```python
from build123d import *

# Parameters (mm, degrees)
SKETCH_1_W               = 764
SKETCH_1_H               = 1500
SKETCH_1_W_2             = 584
SKETCH_1_H_2             = 1320
EXTRUDE_1_DEPTH          = 18
SKETCH_1_3_W             = 28
SKETCH_1_3_H             = 60
EXTRUDE_2_DEPTH          = 18
PATTERN_LINEAR_1_COUNT   = 5
PATTERN_LINEAR_1_PITCH   = 250
MIRROR_1_COPY_1_SKETCH_W = 28
MIRROR_1_COPY_1_SKETCH_H = 60
MIRROR_1_COPY_1_DEPTH    = 18
MIRROR_1_COPY_2_SKETCH_W = 28
MIRROR_1_COPY_2_SKETCH_H = 60
MIRROR_1_COPY_2_DEPTH    = 18
MIRROR_1_COPY_3_SKETCH_W = 28
MIRROR_1_COPY_3_SKETCH_H = 60
MIRROR_1_COPY_3_DEPTH    = 18
MIRROR_1_COPY_4_SKETCH_W = 28
MIRROR_1_COPY_4_SKETCH_H = 60
MIRROR_1_COPY_4_DEPTH    = 18
SKETCH_1_4_W             = 62
SKETCH_1_4_H             = 20
CUT_EXTRUDE_1_DEPTH      = 855.940933632
PATTERN_LINEAR_2_COUNT   = 3
PATTERN_LINEAR_2_PITCH   = 250
MIRROR_2_COPY_1_SKETCH_W = 62
MIRROR_2_COPY_1_SKETCH_H = 20
MIRROR_2_COPY_1_DEPTH    = 855.940933632
MIRROR_2_COPY_2_SKETCH_W = 62
MIRROR_2_COPY_2_SKETCH_H = 20
MIRROR_2_COPY_2_DEPTH    = 855.940933632
FILLET_1_R               = 25
FILLET_2_R               = 25


with BuildPart() as part:
    # 草图1 → 凸台-拉伸1 (new body)
    with BuildSketch(Plane(origin=(0, 0, 0), x_dir=(1, 0, 0), z_dir=(0, 1, 0))):
        Rectangle(SKETCH_1_W, SKETCH_1_H)
        Rectangle(SKETCH_1_W_2, SKETCH_1_H_2, mode=Mode.SUBTRACT)
    extrude(amount=EXTRUDE_1_DEPTH)

    # 草图1<3> → 凸台-拉伸2 (add)
    with BuildSketch(Plane(origin=(0, 0, 0), x_dir=(1, 0, 0), z_dir=(0, 1, 0))):
        with Locations((-396, -500)):
            Rectangle(SKETCH_1_3_W, SKETCH_1_3_H)
    extrude_2 = extrude(amount=EXTRUDE_2_DEPTH)

    # 阵列(线性)1: 凸台-拉伸2 ×5
    with Locations(*[(0, 0, -i * PATTERN_LINEAR_1_PITCH) for i in range(1, PATTERN_LINEAR_1_COUNT)]):
        add(extrude_2)

    # 镜向1: 凸台-拉伸2 across plane
    add(extrude_2.mirror(Plane(origin=(0, 0, 0), x_dir=(0, 0, 1), z_dir=(1, 0, 0))))

    # 镜向1 copy 1 sketch → 镜向1 copy 1 (add)
    with BuildSketch(Plane(origin=(0, 0, -250), x_dir=(-1, 0, 0), z_dir=(0, 1, 0))):
        with Locations((-396, 500)):
            Rectangle(MIRROR_1_COPY_1_SKETCH_W, MIRROR_1_COPY_1_SKETCH_H)
    extrude(amount=MIRROR_1_COPY_1_DEPTH)

    # 镜向1 copy 2 sketch → 镜向1 copy 2 (add)
    with BuildSketch(Plane(origin=(0, 0, -500), x_dir=(-1, 0, 0), z_dir=(0, 1, 0))):
        with Locations((-396, 500)):
            Rectangle(MIRROR_1_COPY_2_SKETCH_W, MIRROR_1_COPY_2_SKETCH_H)
    extrude(amount=MIRROR_1_COPY_2_DEPTH)

    # 镜向1 copy 3 sketch → 镜向1 copy 3 (add)
    with BuildSketch(Plane(origin=(0, 0, -750), x_dir=(-1, 0, 0), z_dir=(0, 1, 0))):
        with Locations((-396, 500)):
            Rectangle(MIRROR_1_COPY_3_SKETCH_W, MIRROR_1_COPY_3_SKETCH_H)
    extrude(amount=MIRROR_1_COPY_3_DEPTH)

    # 镜向1 copy 4 sketch → 镜向1 copy 4 (add)
    with BuildSketch(Plane(origin=(0, 0, -1000), x_dir=(-1, 0, 0), z_dir=(0, 1, 0))):
        with Locations((-396, 500)):
            Rectangle(MIRROR_1_COPY_4_SKETCH_W, MIRROR_1_COPY_4_SKETCH_H)
    extrude(amount=MIRROR_1_COPY_4_DEPTH)

    # 草图1<4> → 切除-拉伸1 (cut, through all)
    with BuildSketch(Plane(origin=(0, 0, 0), x_dir=(1, 0, 0), z_dir=(0, 1, 0))):
        with Locations((-250, -725)):
            Rectangle(SKETCH_1_4_W, SKETCH_1_4_H)
    cut_extrude_1 = extrude(amount=CUT_EXTRUDE_1_DEPTH, mode=Mode.SUBTRACT)

    # 阵列(线性)2: 切除-拉伸1 ×3
    with Locations(*[(i * PATTERN_LINEAR_2_PITCH, 0, 0) for i in range(1, PATTERN_LINEAR_2_COUNT)]):
        add(cut_extrude_1, mode=Mode.SUBTRACT)

    # 镜向2: 切除-拉伸1 across plane
    add(cut_extrude_1.mirror(Plane.XY), mode=Mode.SUBTRACT)

    # 镜向2 copy 1 sketch → 镜向2 copy 1 (cut, through all)
    with BuildSketch(Plane(origin=(250, 0, 0), x_dir=(1, 0, 0), z_dir=(0, 1, 0))):
        with Locations((-250, 725)):
            Rectangle(MIRROR_2_COPY_1_SKETCH_W, MIRROR_2_COPY_1_SKETCH_H)
    extrude(amount=MIRROR_2_COPY_1_DEPTH, mode=Mode.SUBTRACT)

    # 镜向2 copy 2 sketch → 镜向2 copy 2 (cut, through all)
    with BuildSketch(Plane(origin=(500, 0, 0), x_dir=(1, 0, 0), z_dir=(0, 1, 0))):
        with Locations((-250, 725)):
            Rectangle(MIRROR_2_COPY_2_SKETCH_W, MIRROR_2_COPY_2_SKETCH_H)
    extrude(amount=MIRROR_2_COPY_2_DEPTH, mode=Mode.SUBTRACT)

    # 圆角1
    fillet_1_edges = [part.edges().sort_by_distance(p)[0] for p in [
        (-382, 9, -750),
        (-382, 9, 750),
        (382, 9, 750),
        (382, 9, -750),
    ]]
    fillet(fillet_1_edges, radius=FILLET_1_R)

    # 圆角2
    fillet_2_edges = [part.edges().sort_by_distance(p)[0] for p in [
        (292, 9, -660),
        (-292, 9, -660),
        (-292, 9, 660),
        (292, 9, 660),
    ]]
    fillet(fillet_2_edges, radius=FILLET_2_R)


solid = part.part
```
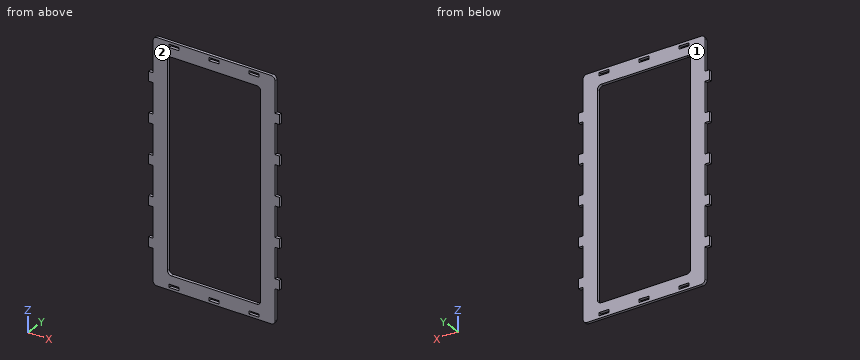
Geometry: final body of the model. Coordinates: model frame, mm. Face numbers are marked on the shaded views. Coordinates: 2 decimals unless noted, no trailing zeros. Order: outer loops, then holes, each group sorted by start corner. A loop starts at its lowest first (then second) coordinate and runs counter-clockwise, first axis right, second up. Notation, with made-up numbers: (-27.5, 21) - (-2.5, 21) arc R22 ccw to (-2.5, 40) - close; hole circle Ø1 at (16, 11). An arc over 180 degrees is marked (long way). Write each question's results on one line, items separated by ' | '.
1) Pull-direction query (Y, two-part tool) for the marked faces 1 and 2; classes: pulls with the +Y half, pulls with the -Y half, needs draft (parallel to the pull), parting line crosses it, or undercut.
Results list:
face 1: pulls with the +Y half | face 2: pulls with the -Y half
2) Section B-B, the plane z = 253. Return loops of the section in (x, y), plus the area to 3 significant figures.
Results list:
outline: (-410, 0) - (-292, 0) - (-292, 18) - (-410, 18) - close; (292, 0) - (410, 0) - (410, 18) - (292, 18) - close | area: 4,250 mm^2
3) Line query: line 1 (X direction, y = 10.5, z = -449); line 2 (Z direction, x = -28, y = 17); line 3 (Z direction, x = 64, y = 4.75). Output: solid intervals per line, ascending. Write a range as from..to.
Results list:
line 1: -382..-292, 292..382 | line 2: -750..-735, -715..-660, 660..715, 735..750 | line 3: -750..-660, 660..750
4) Section A-A, the plane x = -129.5. Return loops of the section in (y, z).
Results list:
outline: (0, -750) - (18, -750) - (18, -660) - (0, -660) - close; (0, 660) - (18, 660) - (18, 750) - (0, 750) - close
5) Pin query (flat end, axial travel): pin 1 (5.5 mm diameter, centred on y = 12.5, z = -372.5, fed in from -X); pin 2 (5.5 mm diameter, centred on y = 7.5, z = 729, fed in from +X); pin 3 (9 mm diameter, centred on x = -396.5, y = 8.5, fed in from -Z). Return the tip coordinate at first contact, or that it passes through.
Results list:
pin 1: x = -382 | pin 2: x = 381.97 | pin 3: z = -530
6) Section C-C, the plane y = 10.5. State how many separate pieces and enclosed holes the cut face has, plus the area to 3 significant figures.
Results list:
separate pieces: 1 | enclosed holes: 7 | area: 384,000 mm^2
